CAD build for the part. Positions are in the model's coordinates, mm. A direction names the side the tool comes from. Coordinates: 2 decimals unless noted, no trailing zeros. Write each loop counter-clockwise with the first axis right and the second up, starting at its lowest first coordinate (ties: lowest second). Pieces come first, ordered by that corner, then holes. Notation, with made-up numbers: M -39.5,30 L -3.5,30 A18 ccw -3.5,55 Z; hole C 14.25,60 d1. An arc over 180 degrees is marked long. Put each result on its own line as item: value. Start each with the question number.
```python
from build123d import *

# Parameters (mm, degrees)
SKETCH1_W           = 116
SKETCH1_H           = 61
BOSS_EXTRUDE1_DEPTH = 3
CHAMFER1_SIZE       = 5
SKETCH2_R           = 1.6
CUT_EXTRUDE1_DEPTH  = 10
SKETCH3_W           = 107
SKETCH3_H           = 52
BOSS_EXTRUDE2_DEPTH = 1
CHAMFER2_SIZE       = 5
SKETCH4_W           = 58.5
SKETCH4_H           = 10
CUT_EXTRUDE2_DEPTH  = 1


with BuildPart() as part:
    # Sketch1 → Boss-Extrude1 (new body)
    with BuildSketch(Plane(origin=(0, 0, 0), x_dir=(1, 0, 0), z_dir=(0, 1, 0))):
        Rectangle(SKETCH1_W, SKETCH1_H)
    extrude(amount=BOSS_EXTRUDE1_DEPTH)

    # Chamfer1
    chamfer1_edges = [part.edges().sort_by_distance(p)[0] for p in [
        (58, 1.5, 30.5),
        (-58, 1.5, 30.5),
        (-58, 1.5, -30.5),
        (58, 1.5, -30.5),
    ]]
    chamfer(chamfer1_edges, length=CHAMFER1_SIZE)

    # Sketch2 → Cut-Extrude1 (cut)
    with BuildSketch(Plane(origin=(0, 3, 0), x_dir=(1, 0, 0), z_dir=(0, 1, 0))):
        with Locations(Location((-53.7, 26.2, 0), (0, 0, 270))):
            Circle(SKETCH2_R)
        with Locations(Location((53.7, 26.2, 0), (0, 0, 270))):
            Circle(SKETCH2_R)
        with Locations(Location((53.7, -26.2, 0), (0, 0, 270))):
            Circle(SKETCH2_R)
        with Locations(Location((-53.7, -26.2, 0), (0, 0, 270))):
            Circle(SKETCH2_R)
    extrude(amount=-CUT_EXTRUDE1_DEPTH, mode=Mode.SUBTRACT)

    # Sketch3 → Boss-Extrude2 (add)
    with BuildSketch(Plane(origin=(0, 3, 0), x_dir=(1, 0, 0), z_dir=(0, 1, 0))):
        Rectangle(SKETCH3_W, SKETCH3_H)
    extrude(amount=BOSS_EXTRUDE2_DEPTH)

    # Chamfer2
    # the kernel refuses this chamfer: 5 mm, written as the material it takes off along each edge
    with BuildSketch(Plane(origin=(53.5, 3, 26), x_dir=(-0.9996219169112968, 0, 0.027495876610586317), z_dir=(0, 1, 0))) as chamfer2_piece_1:
        Polygon((CHAMFER2_SIZE * 0.999621916911, -CHAMFER2_SIZE * 0.0274958766106), (-CHAMFER2_SIZE * 0.0274958766106, -CHAMFER2_SIZE * 0.999621916911), (0, 0), align=None)
    extrude(amount=13.85841494, mode=Mode.SUBTRACT)
    with BuildSketch(Plane(origin=(53.5, 3, -26), x_dir=(-0.9996219169112968, 0, -0.027495876610586282), z_dir=(0, 1, 0)), Plane(origin=(-53.5, 3, -26), x_dir=(-0.027495876610586317, 0, 0.9996219169112968), z_dir=(0, 1, 0)), Plane(origin=(-53.5, 3, 26), x_dir=(0.9996219169112968, 0, 0.027495876610586282), z_dir=(0, 1, 0))) as chamfer2_piece_2:
        Polygon((CHAMFER2_SIZE * 0.999621916911, CHAMFER2_SIZE * 0.0274958766106), (-CHAMFER2_SIZE * 0.0274958766106, CHAMFER2_SIZE * 0.999621916911), (0, 0), align=None)
    extrude(amount=13.85841494, mode=Mode.SUBTRACT)

    # Sketch4 → Cut-Extrude2 (cut)
    with BuildSketch(Plane(origin=(0, 4, 0), x_dir=(1, 0, 0), z_dir=(0, 1, 0))):
        with Locations((0, 21)):
            Rectangle(SKETCH4_W, SKETCH4_H)
    extrude(amount=-CUT_EXTRUDE2_DEPTH, mode=Mode.SUBTRACT)


solid = part.part
```
(1) Two-plate mould, pull along X, no slides. Class faces 5 (the face through (55.05, 1.52, 27.06)), 6 (the face through (55.5, 1.5, -28)), 7 (the face through (-1, 0, 0)): +X half, -X half, draft (parallel to the pull), parting line (faces both ways), or undercut.
(2) Slice it at A-A, the plane x = 32. Write the cut outline in (y, z), then the cut area to 3 significant figures.
(3) Drill centre lines: line 1 (Z direction, x = -53.7, y = 2.1); line 2 (X direction, y = 1.05, z = -26.2); line 3 (X direction, y = 1.45, z = -25). Where is each one in solid material? Low to high. Write a range as [from, to].
(4) Slice it at B-B, the plane z = -10.5. Write the cut outline in (x, y), then the cut area to 3 significant figures.
(5) Which spindle directions (+Z, -Z, +X, -X, +Y, -Y) get a long thin tool onto all of the face, cutting with end or side? Do faces 1 (the face through (-51, 3.5, -23.5)), 2 (the face through (51, 3.5, -23.5)), 3 (the face through (51, 3.5, 23.5)), 4 (the face through (-51, 3.5, 23.5)). Say none if no direction does.
(6) Drop flat-ended pins along their axis: pin 1 (4 mm diameter, centred on x = 53.7, z = -26.2, fed in from +Y); pin 2 (0.5 mm diameter, centred on y = 3.5, z = -22.5, fed in from +X); pin 3 (0.5 mm diameter, centred on x = -21.5, y = 3.5, fed in from +Z). Give the stop position or say it passes through.
Result set:
1. face 5: undercut
1. face 6: +X half
1. face 7: draft
2. outline: M 0,-30.5 L 3,-30.5 L 3,-26 L 4,-26 L 4,26 L 3,26 L 3,30.5 L 0,30.5 Z
2. area: 235 mm^2
3. line 1: z = [-29.8, -27.8], [-24.6, 24.6], [27.8, 29.8]
3. line 2: x = [-57.3, -55.3], [-52.1, 52.1], [55.3, 57.3]
3. line 3: x = [-58, -54.76], [-52.64, 52.64], [54.76, 58]
4. outline: M -58,0 L 58,0 L 58,3 L 53.5,3 L 53.5,4 L -53.5,4 L -53.5,3 L -58,3 Z
4. area: 455 mm^2
5. face 1: -Z, -X, +Y
5. face 2: -Z, +X, +Y
5. face 3: +Z, +X, +Y
5. face 4: +Z, -X, +Y
6. pin 1: stops at y = 3
6. pin 2: stops at x = 52.25
6. pin 3: stops at z = 26
